The listing builds one solid part. Answer for the finished solid, in the listing's coordinates (mm). A direction names the side the tool comes from. Give positions to 0.01 mm unless a question says otherwise; leave off trailing zeros. Order: outer loops, then holes, each group sorted by start corner. A loop starts at its lowest first (then second) coordinate and runs counter-clockwise, first axis right, second up. Notation, with made-up numbers: (22, 81.5) - (40, 81.5) arc R28 ccw to (40, 107.5) - close; hole circle Ø5 at (-5, 42.5). An arc over 180 degrees is marked (long way). Answer in a Markdown table with one row per item.
from build123d import *

# Parameters (mm, degrees)
SKETCH002_W   = 60
SKETCH002_H   = 40
PAD001_DEPTH  = 15
SKETCH003_R   = 4.5
HOLE001_DEPTH = 15.001
SKETCH004_W   = 1.52
SKETCH004_H   = 1.52
POCKET_DEPTH  = 30.001
SKETCH006_R   = 3.3
HOLE003_DEPTH = 15.001


with BuildPart() as part:
    # Sketch002 → Pad001 (new body)
    with BuildSketch(Plane.XZ):
        with Locations((0, 20)):
            Rectangle(SKETCH002_W, SKETCH002_H)
    extrude(amount=PAD001_DEPTH)

    # Sketch003 → Hole001 (cut, through all)
    with BuildSketch(Plane.XZ):
        with Locations((0, 20)):
            Circle(SKETCH003_R)
    extrude(amount=HOLE001_DEPTH, mode=Mode.SUBTRACT)

    # Sketch004 → Pocket (cut, through all)
    with BuildSketch(Plane.YZ):
        with Locations((-0.76, 16.74)):
            Rectangle(SKETCH004_W, SKETCH004_H)
    extrude(amount=POCKET_DEPTH, mode=Mode.SUBTRACT)

    # Sketch006 → Hole003 (cut, through all)
    with BuildSketch(Plane.XZ):
        with Locations((-22.5, 32.5)):
            Circle(SKETCH006_R)
        with Locations((22.5, 32.5)):
            Circle(SKETCH006_R)
        with Locations((22.5, 7.5)):
            Circle(SKETCH006_R)
        with Locations((-22.5, 7.5)):
            Circle(SKETCH006_R)
    extrude(amount=HOLE003_DEPTH, mode=Mode.SUBTRACT)


solid = part.part
Item 1: Determine the mould class of faces 1 (the face through (17, -1, 17.5)), 2 (the face through (0, -7, 40)), 3 (the face through (0, -7, 0)), 4 (the face through (-30, -7, 20)) for opening direction Z: pulls with the +Z half, pulls with the -Z half, needs draft (parallel to the pull), parting line crosses it, or undercut.
Answer block:
| item | result |
|---|---|
| face 1 | undercut |
| face 2 | pulls with the +Z half |
| face 3 | pulls with the -Z half |
| face 4 | needs draft |
Item 2: Which of the six approach directions +Z, -Z, +X, -X, +Y, -Y give full straight-line access (tool end or side, diameter ignored) to faces 5 (the face through (30, -7, 20)), 6 (the face through (16, -1.52, 17))?
Answer block:
| item | result |
|---|---|
| face 5 | +Z, -Z, +X, +Y, -Y |
| face 6 | +X, +Y |
Item 3: Find section C-C on z = 7.5. Write down the section's boundary in (x, y), then the cut area to 3 significant figures.
Answer block:
| item | result |
|---|---|
| outline | (-30, -15) - (-25.8, -15) - (-25.8, 0) - (-30, 0) - close; (-19.2, -15) - (19.2, -15) - (19.2, 0) - (-19.2, 0) - close; (25.8, -15) - (30, -15) - (30, 0) - (25.8, 0) - close |
| area | 702 mm² |
Item 4: Find section D-D on y = -0.75. Write down the section's boundary in (x, z), then the cut area to 3 significant figures.
Answer block:
| item | result |
|---|---|
| outline | (-30, 0) - (30, 0) - (30, 15.98) - (2.02, 15.98) arc R4.5 cw (long way) to (3.74, 17.5) - (30, 17.5) - (30, 40) - (-30, 40) - close; hole circle Ø6.6 at (-22.5, 7.5); hole circle Ø6.6 at (-22.5, 32.5); hole circle Ø6.6 at (22.5, 7.5); hole circle Ø6.6 at (22.5, 32.5) |
| area | 2,160 mm² |
Item 5: Consider line 1 (Z direction, x = 22.5, y = -4.5); line 2 (X direction, y = -9.5, z = 7.5); line 3 (Z direction, x = -20.5, y = -10.5). Determine where each line is inside the solid, lowest interval first.
Answer block:
| item | result |
|---|---|
| line 1 | 0 to 4.2, 10.8 to 29.2, 35.8 to 40 |
| line 2 | -30 to -25.8, -19.2 to 19.2, 25.8 to 30 |
| line 3 | 0 to 4.88, 10.12 to 29.88, 35.12 to 40 |
Item 6: This flat-tipped pin is pushed along its axis until it touches: P1, Ø5.5, axis at x = 22.5, z = 7.5, coming from the -Y side. Where does it stop, or does it pass through?
Answer block:
| item | result |
|---|---|
| P1 | through |
Item 7: Find section A-A on x = 0. Write down the section's boundary in (y, z).
Answer block:
| item | result |
|---|---|
| outline | (-15, 0) - (0, 0) - (0, 15.5) - (-15, 15.5) - close; (-15, 24.5) - (0, 24.5) - (0, 40) - (-15, 40) - close |
Item 8: Find section B-B on x = 22.5. Write down the section's boundary in (y, z).
Answer block:
| item | result |
|---|---|
| outline | (-15, 0) - (0, 0) - (0, 4.2) - (-15, 4.2) - close; (-15, 10.8) - (0, 10.8) - (0, 15.98) - (-1.52, 15.98) - (-1.52, 17.5) - (0, 17.5) - (0, 29.2) - (-15, 29.2) - close; (-15, 35.8) - (0, 35.8) - (0, 40) - (-15, 40) - close |
